```python
from build123d import *

# Parameters (mm, degrees)
SKETCH1_R           = 1.85
BOSS_EXTRUDE1_DEPTH = 78
CHAMFER1_SIZE       = 1


with BuildPart() as part:
    # Sketch1 → Boss-Extrude1 (new body)
    with BuildSketch(Plane.XY):
        with BuildLine():
            Line((41, -10), (-41, -10))
            ThreePointArc((-41, -10), (-43.121320344, -9.121320344), (-44, -7))
            Line((-44, -7), (-44, 7))
            ThreePointArc((-44, 7), (-43.121320344, 9.121320344), (-41, 10))
            Line((-41, 10), (41, 10))
            ThreePointArc((41, 10), (43.121320344, 9.121320344), (44, 7))
            Line((44, 7), (44, -7))
            ThreePointArc((44, -7), (43.121320344, -9.121320344), (41, -10))
        make_face()
        with Locations((-34, 0)):
            Circle(SKETCH1_R, mode=Mode.SUBTRACT)
        with Locations((-17, 0)):
            Circle(SKETCH1_R, mode=Mode.SUBTRACT)
        Circle(SKETCH1_R, mode=Mode.SUBTRACT)
        with Locations((17, 0)):
            Circle(SKETCH1_R, mode=Mode.SUBTRACT)
        with Locations((34, 0)):
            Circle(SKETCH1_R, mode=Mode.SUBTRACT)
    extrude(amount=BOSS_EXTRUDE1_DEPTH)

    # Chamfer1
    chamfer1_edges = [part.edges().sort_by_distance(p)[0] for p in [
        (-35.85, 0, 0),
        (-35.85, 0, 78),
        (-18.85, 0, 0),
        (-18.85, 0, 78),
        (-1.85, 0, 0),
        (-1.85, 0, 78),
        (15.15, 0, 0),
        (15.15, 0, 78),
        (32.15, 0, 0),
        (32.15, 0, 78),
    ]]
    chamfer(chamfer1_edges, length=CHAMFER1_SIZE)


solid = part.part
```
Read the model definition and answer for the solid it produces. Units are mm, in the model's axes. Give positions to 0.01 mm unless a question says otherwise; leave off trailing zeros. Write each loop counter-clockwise with the first axis right and the second up, starting at its lowest first coordinate (ties: lowest second). Pieces come first, ordered by that corner, then holes. Notation, with made-up numbers: (64.5, -28.75) -> (71.5, -28.75) arc R19 cw to (71.5, -12.75) -> close; hole circle Ø4 at (-37.75, -20.75). An arc over 180 degrees is marked (long way). Answer as a JSON object with one key per item and string values.
1) Section C-C on y = 0 is taken. Count the separate pieces of the cut face and the enclosed holes in it, then the cut area to 3 significant figures.
Findings below:
{"separate pieces": "6", "enclosed holes": "0", "area": "5,410 mm^2"}
2) Straight lines are drawn through the part: probe 1 along X at (y, z) = (-0.5, 73.5); probe 2 along Y at (x, z) = (17, 33); probe 3 along Y at (x, z) = (-35.5, 74). For each, find the intervals that lie inside material, in ascending order. Write a range as from..to.
Findings below:
{"probe 1": "x = -44..-35.78, -32.22..-18.78, -15.22..-1.78, 1.78..15.22, 18.78..32.22, 35.78..44", "probe 2": "y = -10..-1.85, 1.85..10", "probe 3": "y = -10..-1.08, 1.08..10"}
3) Section A-A on x = -34 is taken. Write down the section's boundary in (y, z), then the cut area to 3 significant figures.
Findings below:
{"outline": "(-10, 0) -> (-2.85, 0) -> (-1.85, 1) -> (-1.85, 77) -> (-2.85, 78) -> (-10, 78) -> close; (1.85, 1) -> (2.85, 0) -> (10, 0) -> (10, 78) -> (2.85, 78) -> (1.85, 77) -> close", "area": "1,270 mm^2"}
4) Flat-ended cylindrical pins translate along their axes: pin 1 Ø3.5 at (x, y) = (0, 0) entering from +Z; pin 2 Ø5 at (x, y) = (-17, 0) entering from -Z; pin 3 Ø6 at (x, y) = (34, 0) entering from +Z; pin 4 Ø4.5 at (x, y) = (17, 0) entering from -Z. Find the tip coordinate at first contact, or state that the pin passes through.
Findings below:
{"pin 1": "passes through", "pin 2": "stops at z = 0.35", "pin 3": "stops at z = 78", "pin 4": "stops at z = 0.6"}
5) For a pull along Y with two mould halves and no side action, classify faces 1 (the cylindrical face through (-43.1, -9.14, 38.45)), 2 (the cylindrical face through (-15.29, -0.71, 38.47)), 3 (the flat face through (1, 5, 78)) as pulls with the +Y half, pulls with the -Y half, needs draft (parallel to the pull), parting line crosses it, or undercut.
Findings below:
{"face 1": "pulls with the -Y half", "face 2": "undercut", "face 3": "needs draft"}
6) Section B-B on z = 23.5 is taken. Write down the section's boundary in (x, y), then the cut area to 3 significant figures.
Findings below:
{"outline": "(-44, -7) arc R3 ccw to (-41, -10) -> (41, -10) arc R3 ccw to (44, -7) -> (44, 7) arc R3 ccw to (41, 10) -> (-41, 10) arc R3 ccw to (-44, 7) -> close; hole circle Ø3.7 at (-34, 0); hole circle Ø3.7 at (-17, 0); hole circle Ø3.7 at (0, 0); hole circle Ø3.7 at (17, 0); hole circle Ø3.7 at (34, 0)", "area": "1,700 mm^2"}
